Can you work these out from the model? Positions are in its coordinate system, mm. A direction names the side the tool comes from. Coordinates: 2 decimals unless noted, no trailing zeros. Loops run counter-clockwise (first coordinate to the right, second up) from the corner with the lowest first, then second, coordinate; pieces in that order, holes last. Notation, with made-up numbers: (13, 42.5) -> (55, 42.5) arc R10 ccw to (55, 61.5) -> close; hole circle Ø4 at (83.25, -20.75). An arc over 180 degrees is marked (long way). Put each result on its own line as item: value. Start each with the question number.
Item 1: Please list where these lines run through material, in increasing order: L1, parallel to Z at x = 39, y = -16; L2, parallel to Z at x = 9, y = -36.5; L3, parallel to X at y = -14, z = 10.5. Write a range as from..to.
Item 2: We'd pull the mould along Z, two halves only. Please class faces 5 (the flat face through (0, -37, 50)), 6 (the cylindrical face through (0.98, -44.44, 35.24)): pulls with the +Z half, pulls with the -Z half, needs draft (parallel to the pull), parting line crosses it, or undercut.
Item 3: For faces 1 (the cylindrical face through (0.82, -37.44, 0.99)), 2 (the cylindrical face through (-0.02, -39.45, 58.63)), 3 (the cylindrical face through (0.8, -36.19, 19.99)), 4 (the cylindrical face through (0.82, -37.44, 68.49)), which set-ups out of +Z, -Z, +X, -X, +Y, -Y let a thin tool reach every point of the face, with its end or its side?
Item 4: If we section it at B-B on z = 26: Please give me the cut outline in (x, y), plus the area to 3 significant figures.
Item 5: If we section it at A-A on x = 0: Please give me the cut outline in (y, z), plus the area to 3 significant figures.
Item 6: Will these pins go through, and if not, where does the flat tip stop? P1, Ø12, axis at y = -39, z = 39, coming from the -X side; P2, Ø3, axis at y = -24.5, z = 55.5, coming from the +X side; P3, Ø12.5, axis at x = -3, y = -26, coming from the -Z side; P4, Ø1, axis at y = -9.5, z = 30.5, coming from the +X side.
Item 7: If we section it at C-C on x = -34: Please give me the cut outline in (y, z).
```python
from build123d import *

# Parameters (mm, degrees)
REVOLUTION_ANGLE = -180
PAD_DEPTH        = 7.5
PAD001_DEPTH     = 17.5
PAD002_DEPTH     = 17.5


with BuildPart() as part:
    # Sketch → Revolution (revolve)
    with BuildSketch(Plane.XZ):
        Polygon((37.45, 69.5), (37.45, 67.5), (42.45, 67.5), (42.45, 50.0000000001), (36.2, 50.0000000001), (36.2, 48.0000000001), (41.2, 48.0000000001), (41.2, 40.5000000001), (36.2, 40.5000000001), (36.2, 38.5000000001), (42.45, 38.5000000001), (42.45, 21.0000000001), (36.2, 21.0000000001), (36.2, 19.0000000001), (41.2, 19.0000000001), (41.2, 11.5000000001), (36.2, 11.5000000001), (36.2, 9.5000000001), (42.45, 9.5000000001), (42.45, 2.0000000001), (37.45, 2.0000000001), (37.45, 0), (44.45, 0), (44.45, 69.5), align=None)
    revolve(axis=Axis((0, 0, 0), (0, 0, 1)), revolution_arc=REVOLUTION_ANGLE)

    # Sketch001 (on DatumPlane) → Pad (new body)
    with BuildSketch(Plane.XY.offset(2)):
        with BuildLine():
            ThreePointArc((-1.481483635, -42.424140607), (0, -42.45), (1.481483635, -42.424140607))
            Line((1.481483635, -42.424140607), (1.3767851449, -39.4259681259))
            ThreePointArc((-1.3767851449, -39.4259681259), (0, -39.45), (1.3767851449, -39.4259681259))
            Line((-1.3767851449, -39.4259681259), (-1.481483635, -42.424140607))
        make_face()
    extrude(amount=PAD_DEPTH)

    # Sketch002 (on DatumPlane) → Pad001 (join)
    with BuildSketch(Plane.XY.offset(21)):
        with BuildLine():
            ThreePointArc((-1.4815012393, -42.4241399922), (0, -42.45), (1.4815012393, -42.4241399922))
            Line((1.4815012393, -42.4241399922), (1.3768015051, -39.4259675545))
            ThreePointArc((-1.3768015051, -39.4259675545), (0, -39.45), (1.3768015051, -39.4259675545))
            Line((-1.3768015051, -39.4259675545), (-1.4815012393, -42.4241399922))
        make_face()
    extrude(amount=PAD001_DEPTH)

    # Sketch003 (on DatumPlane) → Pad002 (join)
    with BuildSketch(Plane.XY.offset(50)):
        with BuildLine():
            ThreePointArc((-1.4815012393, -42.4241399922), (0, -42.45), (1.4815012393, -42.4241399922))
            Line((1.4815012393, -42.4241399922), (1.3768015051, -39.4259675545))
            ThreePointArc((-1.3768015051, -39.4259675545), (0, -39.45), (1.3768015051, -39.4259675545))
            Line((-1.3768015051, -39.4259675545), (-1.4815012393, -42.4241399922))
        make_face()
    extrude(amount=PAD002_DEPTH)


solid = part.part
```
Solutions:
1. L1: 0..2, 9.5..21, 38.5..50, 67.5..69.5
1. L2: 0..2, 9.5..11.5, 19..21, 38.5..40.5, 48..50, 67.5..69.5
1. L3: -42.19..-33.38, 33.38..42.19
2. face 5: undercut
2. face 6: needs draft
3. face 1: -Z, +Y
3. face 2: +Y
3. face 3: +Z, -Z, +Y
3. face 4: +Z, +Y
4. outline: (-44.45, 0) arc R44.45 ccw to (44.45, 0) -> (42.45, 0) arc R42.45 cw to (1.48, -42.42) -> (1.38, -39.43) arc R39.45 cw to (-1.38, -39.43) -> (-1.48, -42.42) arc R42.45 cw to (-42.45, 0) -> close
4. area: 282 mm^2
5. outline: (-44.45, 0) -> (-37.45, 0) -> (-37.45, 2) -> (-39.45, 2) -> (-39.45, 9.5) -> (-36.2, 9.5) -> (-36.2, 11.5) -> (-41.2, 11.5) -> (-41.2, 19) -> (-36.2, 19) -> (-36.2, 21) -> (-39.45, 21) -> (-39.45, 38.5) -> (-36.2, 38.5) -> (-36.2, 40.5) -> (-41.2, 40.5) -> (-41.2, 48) -> (-36.2, 48) -> (-36.2, 50) -> (-39.45, 50) -> (-39.45, 67.5) -> (-37.45, 67.5) -> (-37.45, 69.5) -> (-44.45, 69.5) -> close
5. area: 355 mm^2
6. P1: x = -29.78
6. P2: x = 38.04
6. P3: through
6. P4: x = 43.53
7. outline: (-28.63, 0) -> (-15.7, 0) -> (-15.7, 2) -> (-25.42, 2) -> (-25.42, 9.5) -> (-12.43, 9.5) -> (-12.43, 11.5) -> (-23.27, 11.5) -> (-23.27, 19) -> (-12.43, 19) -> (-12.43, 21) -> (-25.42, 21) -> (-25.42, 38.5) -> (-12.43, 38.5) -> (-12.43, 40.5) -> (-23.27, 40.5) -> (-23.27, 48) -> (-12.43, 48) -> (-12.43, 50) -> (-25.42, 50) -> (-25.42, 67.5) -> (-15.7, 67.5) -> (-15.7, 69.5) -> (-28.63, 69.5) -> close
